```python
from build123d import *

# Parameters (mm, degrees)
SKETCH_1_R               = 22.5
EXTRUDE_1_DEPTH          = 8
SKETCH_3_R               = 5
EXTRUDE_3_DEPTH          = 8
PATTERN_CIRCULAR_1_COUNT = 15
FILLET_1_R               = 1.5
SKETCH_6_R               = 23
CUT_EXTRUDE_1_DEPTH      = 3


with BuildPart() as part:
    # 草图1 → 凸台-拉伸1 (new body)
    with BuildSketch(Plane(origin=(0, 0, 0), x_dir=(1, 0, 0), z_dir=(0, 1, 0))):
        with Locations(Location((0, 0, 0), (0, 0, 270))):
            Circle(SKETCH_1_R)
    extrude(amount=EXTRUDE_1_DEPTH)

    # 草图3 → 凸台-拉伸3 (add)
    with BuildSketch(Plane(origin=(0, 8, 0), x_dir=(1, 0, 0), z_dir=(0, 1, 0))):
        with Locations((22.5, 0)):
            Circle(SKETCH_3_R)
    extrude_3 = extrude(amount=-EXTRUDE_3_DEPTH)

    # 阵列(圆周)1: 凸台-拉伸3 ×15 about axis
    pattern_circular_1_axis = Axis((0.618008615, 0, 0), (0, 1, 0))
    for i in range(1, PATTERN_CIRCULAR_1_COUNT):
        add(extrude_3.rotate(pattern_circular_1_axis, i * 360 / PATTERN_CIRCULAR_1_COUNT))

    # 圆角1
    fillet_1_edges = [part.edges().sort_by_distance(p)[0] for p in [
        (23.58286781, 4, 4.88133151),
        (23.58286781, 4, -4.88133151),
        (19.612035026, 4, -13.799967965),
        (12.35696252, 4, -20.332464591),
        (3.072118239, 4, -23.349293374),
        (-6.637063891, 4, -22.328817212),
        (-15.091778074, 4, -17.447485702),
        (-20.83012742, 4, -9.549325409),
        (-22.859899195, 4, 0),
        (-20.83012742, 4, 9.549325409),
        (-15.091778074, 4, 17.447485702),
        (-6.637063891, 4, 22.328817212),
        (3.072118239, 4, 23.349293374),
        (12.35696252, 4, 20.332464591),
        (19.612035026, 4, 13.799967965),
    ]]
    fillet(fillet_1_edges, radius=FILLET_1_R)

    # 草图6 → 切除-拉伸1 (cut)
    with BuildSketch(Plane(origin=(0, 8, 0), x_dir=(1, 0, 0), z_dir=(0, 1, 0))):
        with Locations(Location((0, 0, 0), (0, 0, 270))):
            Circle(SKETCH_6_R)
    extrude(amount=-CUT_EXTRUDE_1_DEPTH, mode=Mode.SUBTRACT)


solid = part.part
```
Here's how the part is built. I have some questions about the finished solid (model axes, mm). A direction names the side the tool comes from. Coordinates: 2 decimals unless noted, no trailing zeros. Order: outer loops, then holes, each group sorted by start corner. A loop starts at its lowest first (then second) coordinate and runs counter-clockwise, first axis right, second up.
Item 1: Which directions (+Z, -Z, +X, -X, +Y, -Y) give clear straight access to the entire face, cutting with the end or side of a thin tool? Please do faces 4 (the face through (19.394, 6.521, 12.365)), 5 (the face through (1, 0, 0)).
Response values:
face 4: +Y
face 5: +Z, -Z, +X, -X, -Y
Item 2: Thinking about a two-plate mould opening in Z: for faces 1 (the face through (-25.66, 4.06, -5.66)), 2 (the face through (-12.882, 4.056, 23.246)), 3 (the face through (8.99, 4.056, -25.545)), which applies, pulls with the +Z half, pulls with the -Z half, needs draft (parallel to the pull), parting line crosses it, or undercut?
Response values:
face 1: undercut
face 2: pulls with the +Z half
face 3: pulls with the -Z half
Item 3: I'm going to push a flat-ended pin straight in: pin 1 Ø1.5 at (x, z) = (-14.5, 14.5) entering from +Y. Where does the tip first touch, or does it pass through?
Response values:
pin 1: stops at y = 5
Item 4: If we section it at A-A, the plane x = 0: List the corners of the cut face in (y, z) for me.
Response values:
outline: (0, -26.48) - (8, -26.48) - (8, -23) - (5, -23) - (5, 23) - (8, 23) - (8, 26.48) - (0, 26.48) - close
Item 5: I need wall thicknesses on probe 1 along X at (y, z) = (6.05, 0); probe 2 along Y at (x, z) = (20, -9.5); probe 3 along X at (y, z) = (4.75, -12.5). Which ranges of each line are inside material? Lowest first, please.
Response values:
probe 1: x = -23.93 to -23, 23 to 27.5
probe 2: y = 0 to 5
probe 3: x = -22.07 to 24.08
Item 6: If we section it at B-B, the plane x = 18: List the corners of the cut face in (y, z) for me, then the cut area to 3 significant figures.
Response values:
outline: (0, -20.44) - (8, -20.44) - (8, -14.32) - (5, -14.32) - (5, 14.32) - (8, 14.32) - (8, 20.44) - (0, 20.44) - close
area: 241 mm2
